```python
from build123d import *

# Parameters (mm, degrees)
SKETCH_1_W          = 20
SKETCH_1_H          = 20
SKETCH_1_W_2        = 16
SKETCH_1_H_2        = 16
EXTRUDE_1_DEPTH     = 130
SKETCH_2_R          = 1.65
CUT_EXTRUDE_1_DEPTH = 30
SKETCH_3_R          = 1.65
CUT_EXTRUDE_2_DEPTH = 10


with BuildPart() as part:
    # 草图1 → 凸台-拉伸1 (new body)
    with BuildSketch(Plane.XY):
        Rectangle(SKETCH_1_W, SKETCH_1_H)
        Rectangle(SKETCH_1_W_2, SKETCH_1_H_2, mode=Mode.SUBTRACT)
    extrude(amount=EXTRUDE_1_DEPTH)

    # 草图2 → 切除-拉伸1 (cut)
    with BuildSketch(Plane(origin=(0, 10, 0), x_dir=(1, 0, 0), z_dir=(0, 1, 0))):
        with Locations(Location((0, -120, 0), (0, 0, 270))):
            Circle(SKETCH_2_R)
        with Locations(Location((0, -10, 0), (0, 0, 270))):
            Circle(SKETCH_2_R)
    extrude(amount=-CUT_EXTRUDE_1_DEPTH, mode=Mode.SUBTRACT)

    # 草图3 → 切除-拉伸2 (cut, symmetric)
    with BuildSketch(Plane(origin=(0, 0, 0), x_dir=(0, 0, -1), z_dir=(1, 0, 0))):
        with Locations((-120, 0)):
            Circle(SKETCH_3_R)
        with Locations((-10, 0)):
            Circle(SKETCH_3_R)
    extrude(amount=CUT_EXTRUDE_2_DEPTH, both=True, mode=Mode.SUBTRACT)


solid = part.part
```
Build history of the part. All positions in model axes, mm. A direction names the side the tool comes from. Round coordinates to 2 decimals unless told otherwise and drop trailing zeros. Loops run counter-clockwise (first coordinate to the right, second up) from the corner with the lowest first, then second, coordinate; pieces in that order, holes last.
Item 1: Drill centre lines: line 1 along Z through (x, y) = (0.25, -9); line 2 along Y through (x, z) = (8.65, 120); line 3 along X through (y, z) = (-3.5, 60.5). Where is each one in solid material? Low to high.
Item 2: Which spindle directions (+Z, -Z, +X, -X, +Y, -Y) get a long thin tool onto all of the face, cutting with end or side? Do faces 1 (the face through (-8.986, -0.632, 8.476)), 2 (the face through (-8, 0, 64)). Say none if no direction does.
Item 3: Two-plate mould, pull along X, no slides. Class faces 3 (the face through (-8.986, -0.632, 118.476)), 4 (the face through (-0.632, -8.986, 11.524)), 5 (the face through (-10, 0, 64)), 6 (the face through (0, -8, 64)): released by +X, released by -X, zero draft, split by the parting line, or undercut.
Item 4: Pin check, flat tip, straight feed: P1, Ø6, axis at x = -4, y = 2, coming from the -Z side. Stop position of the tip, or through.
Item 5: Saw through at D-D (x = 0). List the corners of the cut face in (y, z).
Item 6: Saw through at A-A (z = 120). List the corners of the cut face in (x, y).
Item 7: Saw through at C-C (z = 88). List the corners of the cut face in (x, y).
Item 8: Saw through at B-B (y = 5.5). List the corners of the cut face in (x, z).
Worked answers:
1. line 1: z = 0 to 8.37, 11.63 to 118.37, 121.63 to 130
1. line 2: y = -10 to -1.65, 1.65 to 10
1. line 3: x = -10 to -8, 8 to 10
2. face 1: +X, -X
2. face 2: +Z, -Z
3. face 3: zero draft
3. face 4: undercut
3. face 5: released by -X
3. face 6: undercut
4. P1: passes through
5. outline: (-10, 0) - (-8, 0) - (-8, 8.35) - (-10, 8.35) - close; (-10, 11.65) - (-8, 11.65) - (-8, 118.35) - (-10, 118.35) - close; (-10, 121.65) - (-8, 121.65) - (-8, 130) - (-10, 130) - close; (8, 0) - (10, 0) - (10, 8.35) - (8, 8.35) - close; (8, 11.65) - (10, 11.65) - (10, 118.35) - (8, 118.35) - close; (8, 121.65) - (10, 121.65) - (10, 130) - (8, 130) - close
6. outline: (-10, -10) - (-1.65, -10) - (-1.65, -8) - (-8, -8) - (-8, -1.65) - (-10, -1.65) - close; (-10, 1.65) - (-8, 1.65) - (-8, 8) - (-1.65, 8) - (-1.65, 10) - (-10, 10) - close; (1.65, -10) - (10, -10) - (10, -1.65) - (8, -1.65) - (8, -8) - (1.65, -8) - close; (1.65, 8) - (8, 8) - (8, 1.65) - (10, 1.65) - (10, 10) - (1.65, 10) - close
7. outline: (-10, -10) - (10, -10) - (10, 10) - (-10, 10) - close; hole (-8, -8) - (8, -8) - (8, 8) - (-8, 8) - close
8. outline: (-10, 0) - (-8, 0) - (-8, 130) - (-10, 130) - close; (8, 0) - (10, 0) - (10, 130) - (8, 130) - close
